from build123d import *

# Parameters (mm, degrees)
F0_R     = 3.5
F1_DEPTH = 3


with BuildPart() as f1:
    # F0 (on Top) → F1 (new body)
    with BuildSketch(Plane.XY):
        with BuildLine():
            Line((-125.965531, 27.705068), (-143.965531, 27.705068))
            ThreePointArc((-143.965531, 27.705068), (-145.379745, 27.119281), (-145.965531, 25.705068))
            Line((-145.965531, 25.705068), (-145.965531, -70.294932))
            ThreePointArc((-145.965531, -70.294932), (-145.379745, -71.709146), (-143.965531, -72.294932))
            Line((-143.965531, -72.294932), (52.034469, -72.294932))
            ThreePointArc((52.034469, -72.294932), (53.448682, -71.709146), (54.034469, -70.294932))
            Line((54.034469, -70.294932), (54.034469, 25.705068))
            ThreePointArc((54.034469, 25.705068), (53.448682, 27.119281), (52.034469, 27.705068))
            Line((52.034469, 27.705068), (34.034469, 27.705068))
            Line((34.034469, 27.705068), (-15.965531, 27.705068))
            Line((-15.965531, 27.705068), (-75.965531, 27.705068))
            Line((-75.965531, 27.705068), (-125.965531, 27.705068))
        make_face()
        with Locations((-125.965531, -60.294932)):
            Circle(F0_R, mode=Mode.SUBTRACT)
        with Locations((-75.965531, -60.294932)):
            Circle(F0_R, mode=Mode.SUBTRACT)
        with Locations((-15.965531, -60.294932)):
            Circle(F0_R, mode=Mode.SUBTRACT)
        with Locations((34.034469, -60.294932)):
            Circle(F0_R, mode=Mode.SUBTRACT)
        Polygon((-90.965531, -11.294932), (-90.965531, -8.294932), (-0.965531, -8.294932), (-0.965531, -11.294932), (9.434469, -11.294932), (9.434469, -33.294932), (-0.965531, -33.294932), (-0.965531, -36.294932), (-90.965531, -36.294932), (-90.965531, -33.294932), (-101.365531, -33.294932), (-101.365531, -11.294932), align=None, mode=Mode.SUBTRACT)
        with Locations((-125.965531, 15.705068)):
            Circle(F0_R, mode=Mode.SUBTRACT)
        with Locations((-75.965531, 15.705068)):
            Circle(F0_R, mode=Mode.SUBTRACT)
        with Locations((-15.965531, 15.705068)):
            Circle(F0_R, mode=Mode.SUBTRACT)
        with Locations((34.034469, 15.705068)):
            Circle(F0_R, mode=Mode.SUBTRACT)
    extrude(amount=F1_DEPTH)


solid = f1.part
The listing builds one solid part. Answer for the finished solid, in the listing's coordinates (mm). Coordinates: 2 decimals unless noted, no trailing zeros. Write each loop counter-clockwise with the first axis right and the second up, starting at its lowest first coordinate (ties: lowest second). Pieces come first, ordered by that corner, then holes. Notation, with made-up numbers: M 10,67 L 20,67 A13 ccw 20,78 Z; hole C 60,-6 d7. An arc over 180 degrees is marked long. Use one line per item in the form item = value.
Item 1: Find the intervals of material crossed by probe 1 along Y at (x, z) = (6.5, 0.9); probe 2 along Y at (x, z) = (-54, 0.9); probe 3 along X at (y, z) = (-16.5, 2.15), in increasing order.
Model answer:
probe_1 = -72.29 to -33.29, -11.29 to 27.71
probe_2 = -72.29 to -36.29, -8.29 to 27.71
probe_3 = -145.97 to -101.37, 9.43 to 54.03
Item 2: Find section A-A, the plane x = -52. Give the vertices of the cut face in (y, z).
Model answer:
outline = M -72.29,0 L -36.29,0 L -36.29,3 L -72.29,3 Z; M -8.29,0 L 27.71,0 L 27.71,3 L -8.29,3 Z
Item 3: Find section B-B, the plane y = -15. Give the vertices of the cut face in (x, z), plus the area to 3 significant figures.
Model answer:
outline = M -145.97,0 L -101.37,0 L -101.37,3 L -145.97,3 Z; M 9.43,0 L 54.03,0 L 54.03,3 L 9.43,3 Z
area = 268 mm2
Item 4: Find section D-D, the plane x = -16. Give the vertices of the cut face in (y, z), plus the area to 3 significant figures.
Model answer:
outline = M -72.29,0 L -63.79,0 L -63.79,3 L -72.29,3 Z; M -56.8,0 L -36.29,0 L -36.29,3 L -56.8,3 Z; M -8.29,0 L 12.21,0 L 12.21,3 L -8.29,3 Z; M 19.2,0 L 27.71,0 L 27.71,3 L 19.2,3 Z
area = 174 mm2
Item 5: Find section C-C, the plane x = 34. Give the vertices of the cut face in (y, z), plus the area to 3 significant figures.
Model answer:
outline = M -72.29,0 L -63.79,0 L -63.79,3 L -72.29,3 Z; M -56.8,0 L 12.21,0 L 12.21,3 L -56.8,3 Z; M 19.2,0 L 27.71,0 L 27.71,3 L 19.2,3 Z
area = 258 mm2
Item 6: The mould has two halves that part along Y. Classify faces 1 (the face through (-47, 1, 0)), 2 (the face through (-122.732, -61.635, 1.479)), 3 (the face through (-18.545, 18.071, 1.479)): released by +Y, released by -Y, zero draft, split by the parting line, or undercut.
Model answer:
face_1 = zero draft
face_2 = undercut
face_3 = undercut
